Verification items for the finished model (mm, model axes). A direction names the side the tool comes from. Coordinates: 2 decimals unless noted, no trailing zeros. Order: outer loops, then holes, each group sorted by start corner. A loop starts at its lowest first (then second) coordinate and runs counter-clockwise, first axis right, second up. Notation, with made-up numbers: M 72,14.25 L 113,14.25 A29 cw 113,38.25 Z; hole C -11.5,2 d5. An arc over 180 degrees is marked long. Return JSON: item names as keys, results as strings. Group by question number.
1. Mould release check, pull along Z, two halves, no side actions. Record for faces 4 (the flat face through (12, 3, 6.1)), 5 (the cylindrical face through (22.7, 3.5, -0.2)), 6 (the flat face through (-8, 7, 0)): +Z half, -Z half, draft (parallel to the pull), parting line (faces both ways), or undercut.
2. Section check B-B, the plane y = 1.25. Record the cut outline in (x, z).
3. Gauge pin test, flat ends, axial feed: pin 1 (2 mm diameter, centred on x = 12.5, y = 2.5, fed in from -Z); pin 2 (1 mm diameter, centred on x = -8, y = 5.5, fed in from +Z); pin 3 (4 mm diameter, centred on x = 16.5, y = 5.5, fed in from +Z). Record the tip position at first contact, or that the pin passes through.
4. Set-up check for faces 1 (the flat face through (-12, 2.3, 0)), 2 (the flat face through (2.73, 3.45, -13.22)), 3 (the flat face through (6.393, 3.451, 3.007)): record each of +Z, -Z, +X, -X, +Y, -Y from which the full face is reachable in a straight line by a thin tool's end or side.
5. Material ranges on line 1 along Y through (x, z) = (-15, 7.5); line 2 along X through (y, z) = (3, 5); line 3 along Z through (x, y) = (12, 6.25), recorded low to high.
6. Section check C-C, the plane x = -11.7. Record the cut outline in (y, z).
7. Section check D-D, the plane z = -1. Record the cut outline in (x, y).
8. Section check A-A, the plane y = 4. Record the cut outline in (x, z), plus the area to 3 significant figures.
```python
from build123d import *

# Parameters (mm, degrees)
SKETCH1_R           = 12
BOSS_EXTRUDE1_DEPTH = 7
SKETCH1_4_R         = 12
CUT_EXTRUDE1_DEPTH  = 2.3


with BuildPart() as part:
    # Sketch1 → Boss-Extrude1 (new body)
    with BuildSketch(Plane(origin=(0, 0, 0), x_dir=(1, 0, 0), z_dir=(0, 1, 0))):
        with BuildLine():
            ThreePointArc((14.05042735, 10.74595232), (22.7, 0), (14.05042735, -10.74595232))
            Line((14.05042735, -10.74595232), (-8.281196581, -15.630476102))
            ThreePointArc((-8.281196581, -15.630476102), (-27.7, 0), (-8.281196581, 15.630476102))
            Line((-8.281196581, 15.630476102), (14.05042735, 10.74595232))
        make_face()
        with Locations((-11.7, 0)):
            Circle(SKETCH1_R, mode=Mode.SUBTRACT)
        Polygon((15.221836642, -6.1), (18.743673284, 0), (15.221836642, 6.1), (8.178163358, 6.1), (4.656326716, 0), (8.178163358, -6.1), align=None, mode=Mode.SUBTRACT)
        with Locations((-11.7, 0)):
            Circle(SKETCH1_R)
    extrude(amount=BOSS_EXTRUDE1_DEPTH)

    # Sketch1_4 → Cut-Extrude1 (cut)
    with BuildSketch(Plane(origin=(0, 0, 0), x_dir=(1, 0, 0), z_dir=(0, 1, 0))):
        with Locations(Location((-11.7, 0, 0), (0, 0, 270))):  # turned: the seam where the file's is
            Circle(SKETCH1_4_R)
    extrude(amount=CUT_EXTRUDE1_DEPTH, mode=Mode.SUBTRACT)


solid = part.part
```
Answers follow:
{
 "1": {"face 4": "undercut", "face 5": "parting line", "face 6": "draft"},
 "2": {"outline": "M -8.28,-15.63 L 14.05,-10.75 A11 ccw 14.05,10.75 L -8.28,15.63 A16 ccw long Z; hole C -11.7,0 d24; hole M 4.66,0 L 8.18,-6.1 L 15.22,-6.1 L 18.74,0 L 15.22,6.1 L 8.18,6.1 Z"},
 "3": {"pin 1": "z = -11.3", "pin 2": "z = 15.68", "pin 3": "z = 10.64"},
 "4": {"face 1": "-Y", "face 2": "-Z, +X, +Y, -Y", "face 3": "+Y, -Y"},
 "5": {"line 1": "2.3 to 7", "line 2": "-26.9 to 7.54, 15.86 to 21.5", "line 3": "-11.19 to -6.1, 6.1 to 11.19"},
 "6": {"outline": "M 0,-16 L 7,-16 L 7,16 L 0,16 L 0,12 L 2.3,12 L 2.3,-12 L 0,-12 Z"},
 "7": {"outline": "M -27.67,0 L -23.66,0 L -23.66,2.3 L 0.26,2.3 L 0.26,0 L 5.23,0 L 5.23,7 L -27.67,7 Z; M 18.17,0 L 22.65,0 L 22.65,7 L 18.17,7 Z"},
 "8": {"outline": "M -8.28,-15.63 L 14.05,-10.75 A11 ccw 14.05,10.75 L -8.28,15.63 A16 ccw long Z; hole M 4.66,0 L 8.18,-6.1 L 15.22,-6.1 L 18.74,0 L 15.22,6.1 L 8.18,6.1 Z", "area": "1,110 mm^2"}
}
